Job drawing, mm, ordinate dimensions from the low corner. One solid piece. Coordinates: 2 decimals unless noted, no trailing zeros. Write each loop counter-clockwise with the first axis right and the second up, starting at its lowest first coordinate (ties: lowest second). Pieces come first, ordered by that corner, then holes. Notation, with made-up numbers: (12.5, 56.5) - (35.5, 56.5) arc R26 cw to (35.5, 89.5) - close; hole circle Ø8 at (51.5, 49). An arc over 180 degrees is marked (long way). Use one line per item in the form item = value. Start each with the question number.
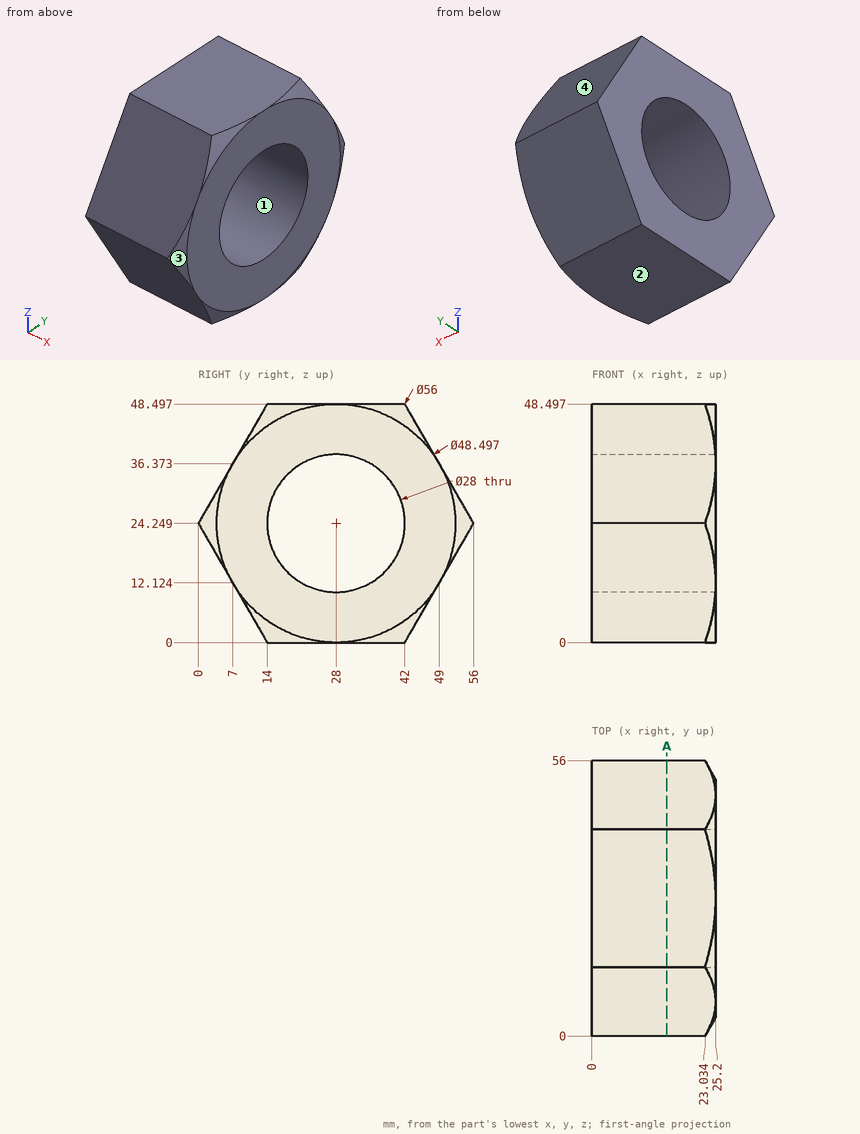
Q1. Slice it at A-A (x = 15.25). List the corners of the cut face in (y, z), plus the area to 3 significant figures.
Q2. Mould opens along Y. For the marked faces 1, 2, 3 and 4 say: released by +Y, released by -Y, zero draft, split by the parting line, or undercut.
Q3. Pin check, flat tips, straight feed: P1, Ø5, axis at x = 20.5, y = 6, coming from the +Z side; P2, Ø12, axis at x = 4.5, z = 16.5, coming from the -Y side; P3, Ø10, axis at x = 15.5, y = 7.5, coming from the +Z side; P4, Ø5, axis at x = 6, y = 24, coming from the -Z side. Stop position of each tip, or through.
Q4. Drill centre lines: probe 1 along Z at (x, y) = (21.5, 29.5); probe 2 along Y at (x, z) = (22.5, 34.5) (1 decimal); probe 3 along Y at (x, z) = (10, 23) (1 decimal). Where is each one in solid material? Low to high.
Solution:
q1.outline = (0, 24.25) - (14, 0) - (42, 0) - (56, 24.25) - (42, 48.5) - (14, 48.5) - close; hole circle Ø28 at (28, 24.25)
q1.area = 1,420 mm2
q2.face_1 = undercut
q2.face_2 = zero draft
q2.face_3 = released by -Y
q2.face_4 = released by +Y
q3.P1 = 38.97
q3.P2 = 1.01
q3.P3 = 45.9
q3.P4 = 0
q4.probe_1 = 0 to 10.33, 38.17 to 48.5
q4.probe_2 = 5.9 to 18.5, 37.5 to 50.1
q4.probe_3 = 0.7 to 14.1, 41.9 to 55.3
